from build123d import *

# Parameters (mm, degrees)
SKETCH2_W           = 250
SKETCH2_H           = 100
BOSS_EXTRUDE1_DEPTH = 50
SKETCH3_W           = 150
SKETCH3_H           = 50
CUT_EXTRUDE1_DEPTH  = 109
SKETCH4_R           = 10
CUT_EXTRUDE2_DEPTH  = 109
SKETCH5_W           = 250
SKETCH5_H           = 50
BOSS_EXTRUDE2_DEPTH = 50
SKETCH8_W           = 150
SKETCH8_H           = 50
BOSS_EXTRUDE3_DEPTH = 50
SKETCH9_W           = 150
SKETCH9_H           = 50
BOSS_EXTRUDE4_DEPTH = 50
SKETCH10_W          = 50
SKETCH10_H          = 250
CUT_EXTRUDE5_DEPTH  = 50
SKETCH11_R          = 10
CUT_EXTRUDE6_DEPTH  = 398


with BuildPart() as part:
    # Sketch2 → Boss-Extrude1 (new body)
    with BuildSketch(Plane(origin=(0, 0, 0), x_dir=(0, 0, -1), z_dir=(1, 0, 0))):
        with Locations((125, 50)):
            Rectangle(SKETCH2_W, SKETCH2_H)
    extrude(amount=BOSS_EXTRUDE1_DEPTH)

    # Sketch3 → Cut-Extrude1 (cut)
    with BuildSketch(Plane(origin=(50, 0, 0), x_dir=(0, 0, -1), z_dir=(1, 0, 0))):
        with Locations((125, 25)):
            Rectangle(SKETCH3_W, SKETCH3_H)
    extrude(amount=-CUT_EXTRUDE1_DEPTH, mode=Mode.SUBTRACT)

    # Sketch4 → Cut-Extrude2 (cut)
    with BuildSketch(Plane(origin=(50, 0, 0), x_dir=(0, 0, -1), z_dir=(1, 0, 0))):
        with Locations((25, 25)):
            Circle(SKETCH4_R)
        with Locations((225, 25)):
            Circle(SKETCH4_R)
    extrude(amount=-CUT_EXTRUDE2_DEPTH, mode=Mode.SUBTRACT)

    # Sketch5 → Boss-Extrude2 (add)
    with BuildSketch(Plane(origin=(50, 0, 0), x_dir=(0, 0, -1), z_dir=(1, 0, 0))):
        with Locations((125, 75)):
            Rectangle(SKETCH5_W, SKETCH5_H)
    boss_extrude2 = extrude(amount=BOSS_EXTRUDE2_DEPTH)

    # Mirror1: Boss-Extrude2 across plane
    add(boss_extrude2.mirror(Plane(origin=(25, 0, 0), x_dir=(0, 0, 1), z_dir=(1, 0, 0))))

    # Sketch8 → Boss-Extrude3 (add)
    with BuildSketch(Plane.XY):
        with Locations((25, 75)):
            Rectangle(SKETCH8_W, SKETCH8_H)
    extrude(amount=BOSS_EXTRUDE3_DEPTH)

    # Sketch9 → Boss-Extrude4 (add)
    with BuildSketch(Plane(origin=(0, 0, -250), x_dir=(-1, 0, 0), z_dir=(0, 0, -1))):
        with Locations((-25, 75)):
            Rectangle(SKETCH9_W, SKETCH9_H)
    extrude(amount=BOSS_EXTRUDE4_DEPTH)

    # Sketch10 → Cut-Extrude5 (cut)
    with BuildSketch(Plane.XZ.offset(-50)):
        with Locations((75, -125)):
            Rectangle(SKETCH10_W, SKETCH10_H)
        with Locations((-25, -125)):
            Rectangle(SKETCH10_W, SKETCH10_H)
    extrude(amount=-CUT_EXTRUDE5_DEPTH, mode=Mode.SUBTRACT)

    # Sketch11 → Cut-Extrude6 (cut)
    with BuildSketch(Plane.XY.offset(50)):
        with Locations((-25, 75)):
            Circle(SKETCH11_R)
        with Locations((75, 75)):
            Circle(SKETCH11_R)
    extrude(amount=-CUT_EXTRUDE6_DEPTH, mode=Mode.SUBTRACT)


solid = part.part
Work out the finished part from the listing and answer in its coordinate system (mm). A direction names the side the tool comes from. Give positions to 0.01 mm unless a question says otherwise; leave off trailing zeros. Order: outer loops, then holes, each group sorted by start corner. A loop starts at its lowest first (then second) coordinate and runs counter-clockwise, first axis right, second up. Notation, with made-up numbers: M 39,-22 L 89,-22 A17 cw 89,1 Z; hole C -9.75,74.25 d3. An arc over 180 degrees is marked long. Return JSON: item names as keys, results as strings.
Q1. Find section D-D, the plane x = 38.5. Write down the section's boundary in (y, z), and give its area (3 significant figures).
Answer below:
{"outline": "M 0,-250 L 50,-250 L 50,-300 L 100,-300 L 100,50 L 50,50 L 50,0 L 0,0 L 0,-50 L 50,-50 L 50,-200 L 0,-200 Z; hole C 25,-225 d20; hole C 25,-25 d20", "area": "21,900 mm^2"}
Q2. The mould has two halves that part along X. Classify faces 1 (the face through (-50, 75, 25)), 2 (the face through (50, 60, -127)), 3 (the face through (-19.62, 83.43, -274.65)), 4 (the face through (64, 75, 0)): pulls with the +X half, pulls with the -X half, needs draft (parallel to the pull), parting line crosses it, or undercut.
Answer below:
{"face 1": "pulls with the -X half", "face 2": "pulls with the +X half", "face 3": "undercut", "face 4": "needs draft"}
Q3. Find section C-C, the plane z = -225. Write down the section's boundary in (x, y), and give its area (3 significant figures).
Answer below:
{"outline": "M 0,0 L 50,0 L 50,15 L 0,15 Z; M 0,35 L 50,35 L 50,100 L 0,100 Z", "area": "4,000 mm^2"}
Q4. Find section A-A, the plane x = -10.5. Write down the section's boundary in (y, z).
Answer below:
{"outline": "M 50,-300 L 100,-300 L 100,-250 L 50,-250 Z; M 50,0 L 100,0 L 100,50 L 50,50 Z"}
Q5. Each of these flat-tipped pins is pushed along its axis until it touches: pin 1 (25 mm diameter, centred on x = -19, y = 68.5, fed in from -Z); pin 2 (15 mm diameter, centred on x = 25.5, y = 13.5, fed in from +Z); pin 3 (25 mm diameter, centred on x = 21, z = 19.5, fed in from -Y); pin 4 (15 mm diameter, centred on x = 17.5, y = 16, fed in from -Z). Where does it stop, or does it pass through?
Answer below:
{"pin 1": "stops at z = -300", "pin 2": "stops at z = 0", "pin 3": "stops at y = 50", "pin 4": "stops at z = -250"}
Q6. Find the intervals of material crossed by line 1 along X through (y, z) = (81, 30); line 2 along Y through (x, z) = (-25, 38.5); line 3 along X through (y, z) = (83, 30.5), in increasing order. Write a range as [from, to].
Answer below:
{"line 1": "x = [-50, -33], [-17, 67], [83, 100]", "line 2": "y = [50, 65], [85, 100]", "line 3": "x = [-50, -31], [-19, 69], [81, 100]"}
Q7. Which of the six approach directions +Z, -Z, +X, -X, +Y, -Y give full straight-line access (tool end or side, diameter ignored) to faces 5 (the face through (64, 75, -250)), 6 (the face through (0, 60, -127)), 7 (the face through (26, 50, 25))?
Answer below:
{"face 5": "+X, +Y, -Y", "face 6": "-X, +Y, -Y", "face 7": "+Z, +X, -X, -Y"}
Q8. Find section B-B, the plane y = 25. Write down the section's boundary in (x, z), and give its area (3 significant figures).
Answer below:
{"outline": "M 0,-250 L 50,-250 L 50,-235 L 0,-235 Z; M 0,-215 L 50,-215 L 50,-200 L 0,-200 Z; M 0,-50 L 50,-50 L 50,-35 L 0,-35 Z; M 0,-15 L 50,-15 L 50,0 L 0,0 Z", "area": "3,000 mm^2"}
